Here's how the part is built. I have some questions about the finished solid (model axes, mm). Face numbers are marked on the shaded views. A direction names the side the tool comes from. Give positions to 0.01 mm unless a question says otherwise; leave off trailing zeros. Write each loop counter-clockwise with the first axis right and the second up, starting at its lowest first coordinate (ties: lowest second). Pieces come first, ordered by that corner, then holes. Notation, with made-up numbers: (33.25, 45.5) - (42.25, 45.5) arc R13 ccw to (42.25, 59.5) - close; hole circle Ø7 at (10.25, 69). An arc over 180 degrees is marked (long way). One line per item, written item: value. Start each with the question number.
1) Imagine slicing it at D-D on y = 11. Write out the boundary of the cut face in (x, z), plus the area to 3 significant figures.
2) Please list where these lines run through material, in increasing order: L1, parallel to X at y = 2.3, z = 5.5; L2, parallel to Y at x = 0, z = -10.1; L3, parallel to Y at x = 0, z = -8. Write a range as [from, to].
3) I'm going to push flat-ended pins straight in: P1, Ø8, axis at x = -9.5, y = 10, coming from the +Z side; P2, Ø6, axis at x = 15.5, y = 7.5, coming from the +Z side; P3, Ø1.8, axis at x = -9, z = -2.5, coming from the +Y side; P4, Ø4, axis at x = 9, z = -2.5, coming from the +Y side. Where does each tip first touch, or does it pass through?
4) Imagine slicing it at B-B on x = 6.5. Write out the boundary of the cut face in (y, z), plus the area to 3 significant figures.
5) On a 3-axis mill with a long thin cutter (end or side, diameter ignored), from which of +Z, -Z, +X, -X, +Y, -Y can I reach the whole of each face in a straight line? I mean the marked faces 1 and 2. Say none if no direction works.
6) Imagine slicing it at A-A on z = -8. Write out the boundary of the cut face in (x, y), plus the area to 3 significant figures.
7) Imagine slicing it at C-C on x = 0.5. Write out the boundary of the cut face in (y, z), plus the area to 3 significant figures.
8) We'd pull the mould along Y, two halves only. Please class the marked faces 3, 4, 5 and 6: +Y half, -Y half, draft (parallel to the pull), parting line (faces both ways), or undercut.
from build123d import *

# Parameters (mm, degrees)
SKETCH_1_W           = 40
SKETCH_1_H           = 20
EXTRUDE_1_DEPTH      = 3
SKETCH_2_W           = 40
SKETCH_2_H           = 3
EXTRUDE_2_DEPTH      = 36
SKETCH_3_R           = 11.5
SKETCH_3_R_2         = 2
CUT_EXTRUDE_M5_DEPTH = 48.010637094
FILLET_1_R           = 12
SKETCH_4_R           = 2
SKETCH_4_R_2         = 11.5
EXTRUDE_3_DEPTH      = 2
SKETCH_5_R           = 3
CUT_EXTRUDE_2_DEPTH  = 2
SKETCH_6_W           = 3
SKETCH_6_H           = 17
EXTRUDE_4_DEPTH      = 20
CUT_EXTRUDE_3_DEPTH  = 58.140178509
SKETCH_8_R           = 1.5
CUT_EXTRUDE_4_DEPTH  = 43.895221179
FILLET_2_R           = 5
FILLET_3_R           = 3


with BuildPart() as part:
    # 草图1 → 凸台-拉伸1 (new body)
    with BuildSketch(Plane(origin=(0, 0, 0), x_dir=(1, 0, 0), z_dir=(0, 1, 0))):
        Rectangle(SKETCH_1_W, SKETCH_1_H)
    extrude(amount=EXTRUDE_1_DEPTH)

    # 草图2 → 凸台-拉伸2 (add)
    with BuildSketch(Plane(origin=(0, 3, 0), x_dir=(1, 0, 0), z_dir=(0, 1, 0))):
        with Locations((0, 8.5)):
            Rectangle(SKETCH_2_W, SKETCH_2_H)
    extrude(amount=EXTRUDE_2_DEPTH)

    # 草图3 → 螺纹-M5 (cut, through all)
    with BuildSketch(Plane.XY.offset(-7)):
        with Locations((0, 24)):
            Circle(SKETCH_3_R)
        with Locations((13.856406461, 32)):
            Circle(SKETCH_3_R_2)
        with Locations((0, 8)):
            Circle(SKETCH_3_R_2)
        with Locations((-13.856406461, 32)):
            Circle(SKETCH_3_R_2)
    extrude(amount=-CUT_EXTRUDE_M5_DEPTH, mode=Mode.SUBTRACT)

    # 圆角1
    fillet_1_edges = [part.edges().sort_by_distance(p)[0] for p in [
        (-20, 39, -8.5),
        (20, 39, -8.5),
    ]]
    fillet(fillet_1_edges, radius=FILLET_1_R)

    # 草图4 → 凸台-拉伸3 (add)
    with BuildSketch(Plane(origin=(0, 0, -10), x_dir=(-1, 0, 0), z_dir=(0, 0, -1))):
        with BuildLine():
            Line((-8, 39), (8, 39))
            ThreePointArc((8, 39), (16.485281374, 35.485281374), (20, 27))
            Line((20, 27), (20, 24))
            ThreePointArc((20, 24), (0, 4), (-20, 24))
            Line((-20, 24), (-20, 27))
            ThreePointArc((-20, 27), (-16.485281374, 35.485281374), (-8, 39))
        make_face()
        with Locations(Location((0, 8, 0), (0, 0, 180))):
            Circle(SKETCH_4_R, mode=Mode.SUBTRACT)
        with Locations(Location((13.856406461, 32, 0), (0, 0, 180))):
            Circle(SKETCH_4_R, mode=Mode.SUBTRACT)
        with Locations(Location((-13.856406461, 32, 0), (0, 0, 180))):
            Circle(SKETCH_4_R, mode=Mode.SUBTRACT)
        with Locations(Location((0, 24, 0), (0, 0, 180))):
            Circle(SKETCH_4_R_2, mode=Mode.SUBTRACT)
    extrude(amount=EXTRUDE_3_DEPTH)

    # 草图5 → 切除-拉伸2 (cut)
    with BuildSketch(Plane(origin=(0, 0, -12), x_dir=(-1, 0, 0), z_dir=(0, 0, -1))):
        with Locations((-15.155444566, 15.25)):
            Circle(SKETCH_5_R)
        with Locations((15.155444566, 15.25)):
            Circle(SKETCH_5_R)
    extrude(amount=-CUT_EXTRUDE_2_DEPTH, mode=Mode.SUBTRACT)

    # 草图6 → 凸台-拉伸4 (add)
    with BuildSketch(Plane(origin=(0, 3, 0), x_dir=(1, 0, 0), z_dir=(0, 1, 0))):
        with Locations((-18.5, -1.5)):
            Rectangle(SKETCH_6_W, SKETCH_6_H)
        with Locations((18.5, -1.5)):
            Rectangle(SKETCH_6_W, SKETCH_6_H)
    extrude(amount=EXTRUDE_4_DEPTH)

    # 草图7 → 切除-拉伸3 (cut, through all)
    with BuildSketch(Plane.ZY.offset(20)):
        Polygon((-7, 23), (10, 3), (10, 23), align=None)
    extrude(amount=-CUT_EXTRUDE_3_DEPTH, mode=Mode.SUBTRACT)

    # 草图8 → 切除-拉伸4 (cut, through all)
    with BuildSketch(Plane(origin=(0, 3, 0), x_dir=(1, 0, 0), z_dir=(0, 1, 0))):
        with Locations(Location((-9, 2.5, 0), (0, 0, 270))):
            Circle(SKETCH_8_R)
        with Locations(Location((9, 2.5, 0), (0, 0, 90))):
            Circle(SKETCH_8_R)
        with Locations(Location((9, -5.5, 0), (0, 0, 270))):
            Circle(SKETCH_8_R)
        with Locations(Location((-9, -5.5, 0), (0, 0, 90))):
            Circle(SKETCH_8_R)
    extrude(amount=-CUT_EXTRUDE_4_DEPTH, mode=Mode.SUBTRACT)

    # 圆角2
    fillet_2_edges = [part.edges().sort_by_distance(p)[0] for p in [
        (-17, 3, 1.5),
        (17, 3, 1.5),
    ]]
    fillet(fillet_2_edges, radius=FILLET_2_R)

    # 圆角3
    fillet_3_edges = [part.edges().sort_by_distance(p)[0] for p in [
        (-18.5, 23, -7),
        (18.5, 23, -7),
    ]]
    fillet(fillet_3_edges, radius=FILLET_3_R)


solid = part.part
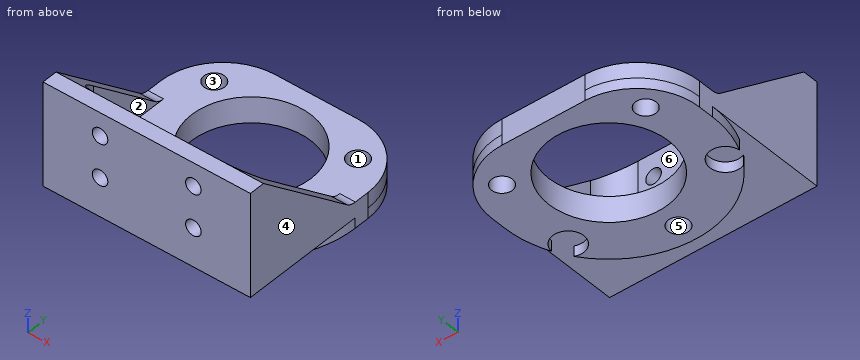
Numbers:
1. outline: (-20, -10) - (-15.2, -10) - (-15.2, -12) - (15.2, -12) - (15.2, -10) - (20, -10) - (20, 3.2) - (17, 3.2) - (17, -7) - (-17, -7) - (-17, 3.2) - (-20, 3.2) - close
1. area: 242 mm^2
2. L1: [-20, -10.5], [-7.5, 7.5], [10.5, 20]
2. L2: [4, 6], [10, 12.5], [35.5, 39]
2. L3: [0, 6], [10, 12.5], [35.5, 39]
3. P1: z = -7
3. P2: z = 8.72
3. P3: through
3. P4: y = 3
4. outline: (0, -10) - (5.09, -10) - (5.09, -12) - (14.51, -12) - (14.51, -7) - (3, -7) - (3, 10) - (0, 10) - close; (33.49, -12) - (39, -12) - (39, -7) - (33.49, -7) - close
4. area: 141 mm^2
5. face 1: +Z, -Z
5. face 2: +Z, +Y
6. outline: (-20, 0) - (20, 0) - (20, 27) arc R12 ccw to (8, 39) - (-8, 39) arc R12 ccw to (-20, 27) - close; hole circle Ø4 at (-13.86, 32); hole circle Ø23 at (0, 24); hole circle Ø4 at (0, 8); hole circle Ø4 at (13.86, 32)
6. area: 1,050 mm^2
7. outline: (0, -10) - (4.01, -10) - (4.01, -12) - (6.06, -12) - (6.06, -7) - (3, -7) - (3, 10) - (0, 10) - close; (9.94, -12) - (12.51, -12) - (12.51, -7) - (9.94, -7) - close; (35.49, -12) - (39, -12) - (39, -7) - (35.49, -7) - close
7. area: 104 mm^2
8. face 3: undercut
8. face 4: draft
8. face 5: undercut
8. face 6: +Y half
